```python
from build123d import *

# Parameters (mm, degrees)
MODEL_R             = 0.95
MODEL_R_2           = 2.5
MODEL_W             = 2
MODEL_H             = 6
MODEL_R_3           = 1.45
BOSS_EXTRUDE2_DEPTH = 5.85


with BuildPart() as part:
    # Model → Boss-Extrude2 (new body)
    with BuildSketch(Plane.XY):
        with BuildLine():
            Line((553.509477136, 560.932469), (545.509477136, 560.932469))
            Line((545.509477136, 560.932469), (545.509477136, 556.356563))
            Line((545.509477136, 556.356563), (546.959477136, 556.356563))
            Line((546.959477136, 556.356563), (546.959477136, 553.956511944))
            Line((546.959477136, 553.956511944), (545.509477136, 553.956511944))
            Line((545.509477136, 553.956511944), (545.509477136, 551.956511944))
            Line((545.509477136, 551.956511944), (542.609477136, 551.956511944))
            Line((542.609477136, 551.956511944), (542.609477136, 553.956511944))
            Line((542.609477136, 553.956511944), (541.159477136, 553.956511944))
            Line((541.159477136, 553.956511944), (541.159477136, 556.356563))
            Line((541.159477136, 556.356563), (542.609477136, 556.356563))
            Line((542.609477136, 556.356563), (542.609477136, 560.932469))
            Line((542.609477136, 560.932469), (540.609477136, 560.932469))
            Line((540.609477136, 560.932469), (540.609477136, 566.932469))
            Line((540.609477136, 566.932469), (537.009477136, 566.932469))
            Line((537.009477136, 566.932469), (537.009477136, 557.932469))
            ThreePointArc((537.009477136, 557.932469), (553.509477136, 541.432469), (570.009477136, 557.932469))
            Line((570.009477136, 557.932469), (570.009477136, 566.932469))
            Line((570.009477136, 566.932469), (566.409477136, 566.932469))
            Line((566.409477136, 566.932469), (566.409477136, 560.932469))
            Line((566.409477136, 560.932469), (564.409477136, 560.932469))
            Line((564.409477136, 560.932469), (564.409477136, 556.356563))
            Line((564.409477136, 556.356563), (565.859477136, 556.356563))
            Line((565.859477136, 556.356563), (565.859477136, 553.956511944))
            Line((565.859477136, 553.956511944), (564.409477136, 553.956511944))
            Line((564.409477136, 553.956511944), (564.409477136, 551.956511944))
            Line((564.409477136, 551.956511944), (561.509477136, 551.956511944))
            Line((561.509477136, 551.956511944), (561.509477136, 553.956511944))
            Line((561.509477136, 553.956511944), (560.059477136, 553.956511944))
            Line((560.059477136, 553.956511944), (560.059477136, 556.356563))
            Line((560.059477136, 556.356563), (561.509477136, 556.356563))
            Line((561.509477136, 556.356563), (561.509477136, 560.932469))
            Line((561.509477136, 560.932469), (553.509477136, 560.932469))
        make_face()
        with Locations((546.609477136, 547.532469)):
            Circle(MODEL_R, mode=Mode.SUBTRACT)
        with Locations((553.509477136, 547.532469)):
            Circle(MODEL_R_2, mode=Mode.SUBTRACT)
        with Locations((560.409477136, 547.532469)):
            Circle(MODEL_R, mode=Mode.SUBTRACT)
        with Locations((549.309477136, 554.532469)):
            Rectangle(MODEL_W, MODEL_H, mode=Mode.SUBTRACT)
        with Locations((553.509477136, 554.532469)):
            Circle(MODEL_R_3, mode=Mode.SUBTRACT)
        with Locations((557.709477136, 554.532469)):
            Rectangle(MODEL_W, MODEL_H, mode=Mode.SUBTRACT)
    extrude(amount=BOSS_EXTRUDE2_DEPTH)


solid = part.part
```
Read the model definition and answer for the solid it produces. Units are mm, in the model's axes. A direction names the side the tool comes from. Round coordinates to 2 decimals unless told otherwise and drop trailing zeros. Write each loop counter-clockwise with the first axis right and the second up, starting at its lowest first coordinate (ties: lowest second). Pieces come first, ordered by that corner, then holes. Notation, with made-up numbers: (-2, 69) - (32, 69) arc R18 ccw to (32, 82) - close; hole circle Ø11 at (-1.5, -37). An arc over 180 degrees is marked (long way). One line per item, written item: value.
Q1. Which of the six approach directions +Z, -Z, +X, -X, +Y, -Y give full straight-line access (tool end or side, diameter ignored) to faces 4 (the flat face through (540.609, 564, 3)), 5 (the flat face through (546.959, 555, 3)), 6 (the flat face through (553, 552, 0))?
The answers:
face 4: +Z, -Z, +Y
face 5: +Z, -Z
face 6: -Z, +X, -X, +Y, -Y
Q2. Straight lines are drawn through the part: line 1 (X direction, y = 557.75, z = 1.4); line 2 (X direction, y = 562, z = 1.1); line 3 (X direction, y = 556.75, z = 4.5). For each, find the intervals that lie inside material, in ascending order. Write a range as from..to.
The answers:
line 1: x = 537.01..542.61, 545.51..561.51, 564.41..570.01
line 2: x = 537.01..540.61, 566.41..570.01
line 3: x = 537.05..542.61, 545.51..548.31, 550.31..556.71, 558.71..561.51, 564.41..569.97
Q3. Each of these flat-tipped pins is pushed along its axis until it touches: P1, Ø3, axis at y = 556, z = 5, coming from the -X side; P2, Ø6, axis at x = 541, y = 562.5, coming from the -Z side; P3, Ø0.6, axis at y = 553, z = 2, coming from the -X side; P4, Ø2, axis at x = 564.5, z = 4, coming from the -Y side. Where does it stop, or does it pass through?
The answers:
P1: stops at x = 537.02
P2: stops at z = 0
P3: stops at x = 537.67
P4: stops at y = 544.8
Q4. Find section B-B (x = 546). Determine the outline of the cut face in (y, z), and give its area (3 significant figures).
The answers:
outline: (543.24, 0) - (546.8, 0) - (546.8, 5.85) - (543.24, 5.85) - close; (548.26, 0) - (553.96, 0) - (553.96, 5.85) - (548.26, 5.85) - close; (556.36, 0) - (560.93, 0) - (560.93, 5.85) - (556.36, 5.85) - close
area: 80.9 mm2
Q5. Find section D-D (x = 567.5). Determine the outline of the cut face in (y, z).
The answers:
outline: (549.19, 0) - (566.93, 0) - (566.93, 5.85) - (549.19, 5.85) - close
Q6. Find section C-C (z = 4). Count the separate pieces of the cut face and the enclosed holes in it, and give its area (3 significant figures).
The answers:
separate pieces: 1
enclosed holes: 6
area: 448 mm2
Q7. For a pull along X with two mould halves and no side action, classify faces 1 (the flat face through (561.509, 553, 3)), 2 (the flat face through (553, 552, 5.85)), 3 (the flat face through (565, 553.957, 3)) as pulls with the +X half, pulls with the -X half, needs draft (parallel to the pull), parting line crosses it, or undercut.
The answers:
face 1: undercut
face 2: needs draft
face 3: undercut
Q8. Find section A-A (y = 560.5). Determine the outline of the cut face in (x, z).
The answers:
outline: (537.01, 0) - (542.61, 0) - (542.61, 5.85) - (537.01, 5.85) - close; (545.51, 0) - (561.51, 0) - (561.51, 5.85) - (545.51, 5.85) - close; (564.41, 0) - (570.01, 0) - (570.01, 5.85) - (564.41, 5.85) - close
